Source: CAD feature listing. Evaluate the final solid. Frame: model axes, mm. A direction names the side the tool comes from. Coordinates: 2 decimals unless noted, no trailing zeros. Loops run counter-clockwise (first coordinate to the right, second up) from the corner with the lowest first, then second, coordinate; pieces in that order, holes last. Notation, with made-up numbers: (-36.75, 33) -> (14.25, 33) arc R18 cw to (14.25, 37) -> close; hole circle Ø7 at (45, 67.25). An arc over 180 degrees is marked (long way). Answer as a JSON object with one key per item and string values. Group by question number.
from build123d import *

# Parameters (mm, degrees)
SKETCH4_R           = 4.7625
BOSS_EXTRUDE2_DEPTH = 6.35


with BuildPart() as part:
    # Sketch4 → Boss-Extrude2 (new body)
    with BuildSketch(Plane.XY):
        with BuildLine():
            Line((0, 0), (0, 19.05))
            ThreePointArc((0, 19.05), (1.859871939, 23.540128061), (6.35, 25.4))
            Line((6.35, 25.4), (82.55, 25.4))
            ThreePointArc((82.55, 25.4), (87.040128061, 23.540128061), (88.9, 19.05))
            Line((88.9, 19.05), (88.9, -25.4))
            Line((88.9, -25.4), (69.85, -25.4))
            Line((69.85, -25.4), (69.85, -6.35))
            ThreePointArc((69.85, -6.35), (67.990128061, -1.859871939), (63.5, 0))
            Line((63.5, 0), (0, 0))
        make_face()
        with Locations((12.7, 12.7)):
            Circle(SKETCH4_R, mode=Mode.SUBTRACT)
    extrude(amount=BOSS_EXTRUDE2_DEPTH)


solid = part.part
1. Ray query, L1, parallel to Y at x = 12.7, z = 2.75; L2, parallel to Y at x = 33.5, z = 2.5; L3, parallel to X at y = -15, z = 1.5. Return the intervals inside material, ascending.
2. Reachability of faces 1 (the face through (32, 0, 3)), 2 (the face through (55, 6, 6.35)) from +Z, -Z, +X, -X, +Y, -Y: full face, straight path, thin tool, end or side. Return the list, or none.
3. Section query B-B on x = 12.7. Return loops of the section in (y, z), then the cut area to 3 significant figures.
4. Section query D-D on x = 43. Return loops of the section in (y, z), then the cut area to 3 significant figures.
5. Mould query, pull axis Y, two halves, no side actions, for faces 3 (the face through (0, 9, 3)), 4 (the face through (86.99, 23.59, 3.13)), 5 (the face through (68.04, -1.91, 3.13)), 6 (the face through (7.942, 12.909, 3.131)). Classes: pulls with the +Y half, pulls with the -Y half, needs draft (parallel to the pull), parting line crosses it, or undercut.
6. Pin query (flat end, axial travel): pin 1 Ø3 at (y, z) = (-20, 3) entering from -X; pin 2 Ø2 at (x, z) = (50.5, 4) entering from -Y. Return the tip coordinate at first contact, or that it passes through.
7. Section query A-A on y = 12.7. Return loops of the section in (x, z), then the cut area to 3 significant figures.
Solved:
{
 "1": {"L1": "0 to 7.94, 17.46 to 25.4", "L2": "0 to 25.4", "L3": "69.85 to 88.9"},
 "2": {"face 1": "+Z, -Z, -X, -Y", "face 2": "+Z, +X, -X, +Y, -Y"},
 "3": {"outline": "(0, 0) -> (7.94, 0) -> (7.94, 6.35) -> (0, 6.35) -> close; (17.46, 0) -> (25.4, 0) -> (25.4, 6.35) -> (17.46, 6.35) -> close", "area": "101 mm^2"},
 "4": {"outline": "(0, 0) -> (25.4, 0) -> (25.4, 6.35) -> (0, 6.35) -> close", "area": "161 mm^2"},
 "5": {"face 3": "needs draft", "face 4": "pulls with the +Y half", "face 5": "pulls with the -Y half", "face 6": "undercut"},
 "6": {"pin 1": "x = 69.85", "pin 2": "y = 0"},
 "7": {"outline": "(0, 0) -> (7.94, 0) -> (7.94, 6.35) -> (0, 6.35) -> close; (17.46, 0) -> (88.9, 0) -> (88.9, 6.35) -> (17.46, 6.35) -> close", "area": "504 mm^2"}
}
